Autodesk Inventor part; units mm, degrees
ref_plane "YZ Plane" through (0, 0, 0) normal (1, 0, 0) x (0, 1, 0)
ref_plane "XZ Plane" through (0, 0, 0) normal (0, 1, 0) x (-1, 0, 0)
ref_plane "XY Plane" through (0, 0, 0) normal (0, 0, 1) x (1, 0, 0)
sketch "草圖1" plane through (0, 0, 0) normal (0, 1, 0) x (-1, 0, 0)
  line L0 (-33.5, 27) -> (33.5, 27)
  line L1 (33.5, 27) -> (33.5, -27)
  line L2 (33.5, -27) -> (-33.5, -27)
  line L3 (-33.5, -27) -> (-33.5, 27)
  line L4 (-33.5, 27) -> (33.5, -27) construction
  line L5 (33.5, 27) -> (-33.5, -27) construction
  line L6 (43.5, -4.5) -> (33.5, -4.5)
  line L7 (33.5, -4.5) -> (33.5, 4.5)
  line L8 (33.5, 4.5) -> (43.5, 4.5)
  line L9 (43.5, 4.5) -> (43.5, -4.5)
  line L10 (-33.5, -4.5) -> (-43.5, -4.5)
  line L11 (-43.5, -4.5) -> (-43.5, 4.5)
  line L12 (-43.5, 4.5) -> (-33.5, 4.5)
  line L13 (-33.5, 4.5) -> (-33.5, -4.5)
  point P0 (0, 0)
  point P1 (33.5, 0)
  point P2 (-33.5, 0)
  point P3 (-33.5, 4.5)
  point P4 (-33.5, -4.5)
  dimension "d0" = 67
  dimension "d1" = 54
  dimension "d2" = 9
  dimension "d3" = 10
extrude "擠出1" add sketch "草圖1" along normal blind 100
sketch "草圖2" plane through (-33.5, 0, 27) normal (0, 0, 1) x (1, 0, 0)
  circle A0 centre (33.5, 33) radius 30
  line L0 (0, 0) -> (67, 0)
  line L1 (3.5, 33) -> (63.5, 33)
  line L2 (63.5, 33) -> (63.5, -12.4903)
  line L3 (63.5, -12.4903) -> (3.5, -12.4903)
  line L4 (3.5, -12.4903) -> (3.5, 33)
  point P0 (33.5, 0)
  point P1 (33.5, 0)
  point P2 (63.5, 33)
  dimension "d6" = 33
  dimension "d7" = 60
extrude "擠出2" cut sketch "草圖2" against normal through all
sketch "草圖3" plane through (33.5, 100, -27) normal (0, 0, -1) x (-1, 0, 0)
  line L0 (3.5, -100) -> (3.5, -67)
  arc A0 (63.5, -67) -> (3.5, -67) centre (33.5, -67) ccw
  line L1 (63.5, -67) -> (63.5, -100)
  line L2 (63.5, -100) -> (67, -100)
  line L3 (67, -100) -> (67, 0)
  line L4 (0, 0) -> (67, 0)
  line L5 (0, -100) -> (0, 0)
  line L6 (0, -100) -> (3.5, -100)
  line L7 (63.5, -67) -> (63.5, -100)
  line L8 (63.5, -100) -> (3.5, -100)
  point P0 (33.5, -100)
sketch "草圖4" plane through (-33.5, 100, 27) normal (0, 0, 1) x (1, 0, 0)
  circle A0 centre (33.5, -65) radius 30
  arc A1 (63.5, -67) -> (3.5, -67) centre (33.5, -67) ccw construction
  line L0 (63.5, -100) -> (3.5, -100)
  line L1 (3.5, -100) -> (3.5, -65)
  line L2 (3.5, -65) -> (63.5, -65)
  line L3 (63.5, -65) -> (63.5, -100)
  point P0 (33.5, -100)
  dimension "d10" = 60
  dimension "d11" = 2
loft "斷面混成1" cut profiles "草圖3", "草圖4" contours L0 A0 L1 L8 / all
properties part number "Slider-1"
Design review of the part built by this model. Coordinates are the model's own, in mm. A direction names the side the tool comes from. Give positions to 0.01 mm unless a question says otherwise; leave off trailing zeros. Write each loop counter-clockwise with the first axis right and the second up, starting at its lowest first coordinate (ties: lowest second). Pieces come first, ordered by that corner, then holes. Notation, with made-up numbers: M 69,20 L 93,20 A11 cw 93,39 Z; hole C 16,17 d2. An arc over 180 degrees is marked long. Answer as a JSON object with one key per item and string values. Group by question number.
1) We need section B-B (y = 85.5). Give the boundary of the cut face in (x, z).
2) We need section A-A (y = 28.5). Give the boundary of the cut face in (x, z).
3) Tool access review of faces 1 (the face through (-33.5, 49, -16)), 2 (the face through (33.5, 49, -16)), 3 (the face through (-33.5, 49, 16)): name each direction out of +Z, -Z, +X, -X, +Y, -Y from which nothing blocks a thin tool from reaching the whole face with its end or side.
4) We need section C-C (x = -37). Give the boundary of the cut face in (y, z), and give its area (3 significant figures).
5) Clearance check with flat-ended pins moving along their axes: pin 1 Ø1.5 at (y, z) = (77.5, 9.5) entering from -X; pin 2 Ø10 at (y, z) = (30.5, 5) entering from -X; pin 3 Ø7 at (y, z) = (48.5, 15.5) entering from +X; pin 4 Ø8 at (x, y) = (-39.5, 39.5) entering from +Z. State where each tip first meets the part, or that it passes through.
6) For line 1 along X through (y, z) = (13, 5); line 2 along X through (y, z) = (64.5, 8.5); line 3 along Z through (x, y) = (-35.5, 68), list the stretches that pass through material, from the lowest coordinate up.
Answer key:
{
 "1": {"outline": "M -43.5,-4.5 L -33.5,-4.5 L -33.5,-27 L 33.5,-27 L 33.5,-4.5 L 43.5,-4.5 L 43.5,4.5 L 33.5,4.5 L 33.5,27 L -33.5,27 L -33.5,4.5 L -43.5,4.5 Z"},
 "2": {"outline": "M -43.5,-4.5 L -33.5,-4.5 L -33.5,-27 L -30,-27 L -30,27 L -33.5,27 L -33.5,4.5 L -43.5,4.5 Z; M 30,-27 L 33.5,-27 L 33.5,-4.5 L 43.5,-4.5 L 43.5,4.5 L 33.5,4.5 L 33.5,27 L 30,27 Z"},
 "3": {"face 1": "-Z, -X, +Y, -Y", "face 2": "-Z, +X, +Y, -Y", "face 3": "+Z, -X, +Y, -Y"},
 "4": {"outline": "M 0,-4.5 L 100,-4.5 L 100,4.5 L 0,4.5 Z", "area": "900 mm²"},
 "5": {"pin 1": "stops at x = -33.5", "pin 2": "stops at x = -43.5", "pin 3": "stops at x = 33.5", "pin 4": "stops at z = 4.5"},
 "6": {"line 1": "x = -33.5 to -30, 30 to 33.5", "line 2": "x = -33.5 to 33.5", "line 3": "z = -4.5 to 4.5"}
}
